For this review, use the dimensioned drawing (mm, ordinates from the lowest corner) and the shaded views. Give positions to 0.01 mm unless a question says otherwise; leave off trailing zeros. Order: outer loops, then holes, each group sorted by start corner. A loop starts at its lowest first (then second) coordinate and runs counter-clockwise, first axis right, second up.
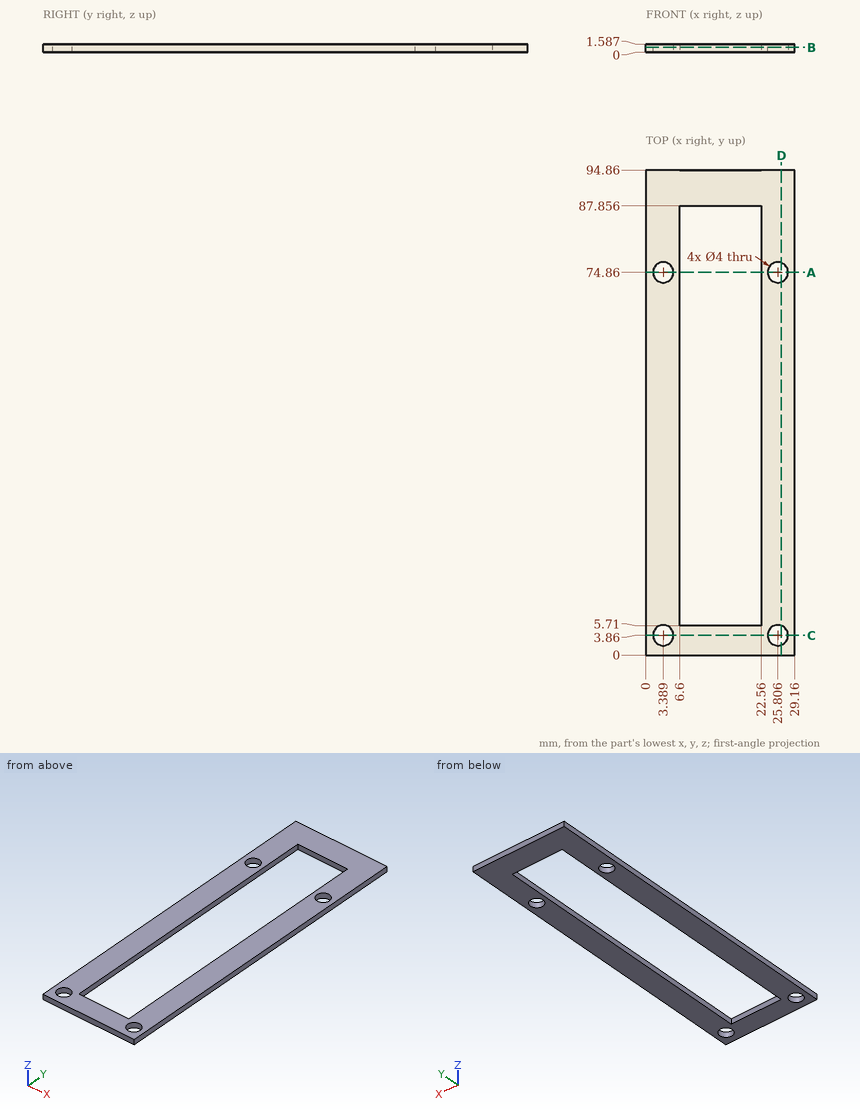
1. Take a section at D-D (x = 26.5). State the section outline as (y, z) points (1 decimal).
Recorded:
outline: (0, 0) - (2, 0) - (2, 1.6) - (0, 1.6) - close; (5.7, 0) - (73, 0) - (73, 1.6) - (5.7, 1.6) - close; (76.7, 0) - (94.9, 0) - (94.9, 1.6) - (76.7, 1.6) - close
2. Take a section at B-B (z = 0.95). State the section outline as (x, y) points (1 decimal).
Recorded:
outline: (0, 0) - (29.2, 0) - (29.2, 94.9) - (0, 94.9) - close; hole circle Ø4 at (3.4, 3.9); hole circle Ø4 at (3.4, 74.9); hole (6.6, 5.7) - (22.6, 5.7) - (22.6, 87.9) - (6.6, 87.9) - close; hole circle Ø4 at (25.8, 3.9); hole circle Ø4 at (25.8, 74.9)
3. For pin 1 (6.5 mm diameter, centred on x = 25.81, y = 3.86, fed in from -Z); pin 2 (3 mm diameter, centred on x = 3.39, y = 3.86, fed in from -Z), all flat-tipped, find the tip position at first contact; note any pin that passes through.
Recorded:
pin 1: stops at z = 0
pin 2: passes through
4. Take a section at C-C (y = 3.86). State the section outline as (x, z) points (1 decimal).
Recorded:
outline: (0, 0) - (1.4, 0) - (1.4, 1.6) - (0, 1.6) - close; (5.4, 0) - (23.8, 0) - (23.8, 1.6) - (5.4, 1.6) - close; (27.8, 0) - (29.2, 0) - (29.2, 1.6) - (27.8, 1.6) - close
5. For line 1 along X through (y, z) = (23, 0.5); line 2 along Y through (x, z) = (8.75, 0.6); line 3 along Y through (x, z) = (24.25, 0.45) (1 decimal), list the stretches that pass through material, from the lowest coordinate up.
Recorded:
line 1: x = 0 to 6.6, 22.56 to 29.16
line 2: y = 0 to 5.71, 87.86 to 94.86
line 3: y = 0 to 2.6, 5.1 to 73.6, 76.1 to 94.9
6. Take a section at A-A (y = 74.86). State the section outline as (x, z) points (1 decimal).
Recorded:
outline: (0, 0) - (1.4, 0) - (1.4, 1.6) - (0, 1.6) - close; (5.4, 0) - (6.6, 0) - (6.6, 1.6) - (5.4, 1.6) - close; (22.6, 0) - (23.8, 0) - (23.8, 1.6) - (22.6, 1.6) - close; (27.8, 0) - (29.2, 0) - (29.2, 1.6) - (27.8, 1.6) - close
